Work out the finished part from the listing and answer in its coordinate system (mm). Round coordinates to 2 decimals unless told otherwise and drop trailing zeros. Loops run counter-clockwise (first coordinate to the right, second up) from the corner with the lowest first, then second, coordinate; pieces in that order, holes last. Notation, with made-up numbers: M 42.25,-4.5 L 80.25,-4.5 A18 cw 80.25,5.5 Z; hole C -39.75,-11.5 d11. An arc over 180 degrees is marked long. One line per item, written item: value.
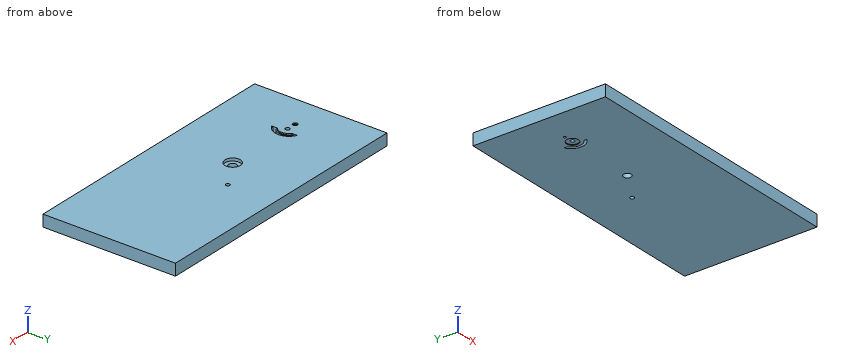
Autodesk Inventor part; units mm, degrees
ref_plane "Plano de trabajo1" through (-95, 0, 0) normal (0, 0, -1) x (-1, 0, 0)
ref_plane "YZ Plane" through (0, 0, 0) normal (1, 0, 0) x (0, 1, 0)
ref_plane "XZ Plane" through (0, 0, 0) normal (0, 1, 0) x (-1, 0, 0)
sketch "Boceto2" plane through (0, 0, 0) normal (0, 0, 1) x (1, 0, 0)
  line L0 (130, -85) -> (-130, -85)
  line L1 (-130, -85) -> (-130, 85)
  line L2 (-130, 85) -> (130, 85)
  line L3 (130, 85) -> (130, -85)
  line L4 (130, -85) -> (-130, 85) construction
  line L5 (-130, -85) -> (130, 85) construction
  point P0 (0, 0)
  dimension "d0" = 260
  dimension "d1" = 170
extrude "Extrusión1" add sketch "Boceto2" along normal blind 15
sketch "Boceto3" plane through (0, 0, 15) normal (0, 0, 1) x (1, 0, 0)
  line L0 (-95, 0) -> (-4.19, 0) construction
  circle A0 centre (-95, 0) radius 2.625
  circle A1 centre (-4.19, 0) radius 9.875
  line L1 (-130, 85) -> (-130, -85)
  line L2 (130, -85) -> (130, 85)
  line L3 (-130, -85) -> (130, -85)
  line L4 (130, 0) -> (80, 0) construction
  line L5 (80, 0) -> (80, -23.2237) construction
  arc A2 (-102.5, -15.9496) -> (-102.5, 15.9496) centre (-109.9995, 0) ccw
  arc A3 (-102.5, -9.8973) -> (-102.5, 9.8973) centre (-109.9995, 0) ccw
  line L6 (-95, 0) -> (-102.5, 0)
  line L7 (-102.5, 15.9496) -> (-102.5, 12.8966)
  line L8 (-102.5, 15.9496) -> (-102.5, 9.8973)
  line L9 (-102.5, -9.8973) -> (-102.5, -15.9496)
  point P0 (0, 0)
  point P1 (-130, 0)
  point P2 (-92.375, 0)
  point P3 (-97.5893, -0.4312)
  point P4 (-97.5893, 0.4312)
  dimension "d7" = 5.25
  dimension "d8" = 19.75
  dimension "d14" = 85
  dimension "d29" = 50
  dimension "d31" = 35
  dimension "d32" = 134.19
  dimension "d139" = 125.81
  dimension "d141" = 7.5
sketch "Boceto5" plane through (0, 0, 0) normal (0, 0, -1) x (-1, 0, 0)
  line L0 (-130, -85) -> (-130, 85)
  line L1 (130, -85) -> (-130, -85)
  line L2 (-130, -85) -> (-130, 85)
  line L3 (-130, 85) -> (130, 85)
  line L4 (130, 85) -> (130, -85)
  line L5 (130, -85) -> (-130, 85) construction
  line L6 (-130, -85) -> (130, 85) construction
  line L7 (119.5, 74.5) -> (-119.5, 74.5)
  line L8 (-119.5, 74.5) -> (-119.5, -74.5)
  line L9 (-119.5, -74.5) -> (119.5, -74.5)
  line L10 (119.5, -74.5) -> (119.5, 74.5)
  circle A0 centre (95, 0) radius 2.625
  circle A1 centre (95, 0) radius 2.625
  point P0 (0, 0)
  dimension "d23" = 10.5
  dimension "d25" = 5.25
sketch "Boceto6" plane through (0, 0, 15) normal (0, 0, 1) x (1, 0, 0)
  circle A0 centre (-4.19, 0) radius 10.125
  line L0 (-4.19, 0) -> (35.81, 0)
  line L1 (35.81, 0) -> (35.81, 25)
  circle A1 centre (35.81, 25) radius 2.5
  point P0 (0, 0)
  dimension "d35" = 40
  dimension "d36" = 25
  dimension "d152" = 5
ref_plane "Plano de trabajo4" through (0, 0, -4) normal (0, 0, -1) x (-1, 0, 0)
sketch "Boceto10" plane through (0, 0, -4) normal (0, 0, -1) x (-1, 0, 0)
  circle A0 centre (95, 0) radius 2.625
  circle A1 centre (95, 0) radius 7.5
  point P0 (0, 0)
  dimension "d51" = 15
ref_plane "Plano de trabajo1" through (-95, 0, 0) normal (0, 0, -1) x (-1, 0, 0)
sketch "Boceto12" plane through (0, 0, 15) normal (0, 0, 1) x (1, 0, 0)
  circle A0 centre (-95, 0) radius 2.625 construction
  circle A1 centre (-95, 0) radius 7.5 construction
  line L0 (-95, 0) -> (-82.5, 0) construction
  circle A2 centre (-82.5, 0) radius 3
  line L1 (-95, 0) -> (-107.5, 0) construction
  circle A3 centre (-107.5, 0) radius 3
  circle A4 centre (-107.5, 0) radius 1.5 construction
  circle A5 centre (-82.5, 0) radius 1.5 construction
  line L2 (-82.5, 0) -> (-97.5, 0) construction
  line L3 (-97.5, 0) -> (-97.5, 18.5) construction
  arc A6 (-89.1168, -15.9286) -> (-89.9998, 16.363) centre (-97.5, 0) ccw
  arc A7 (-89.9998, -16.2295) -> (-89.1168, -15.9286) centre (-90.514, -13.2739) ccw
  arc A8 (-89.9998, -16.2295) -> (-89.1168, -15.9286) centre (-90.514, -13.2739) ccw
  arc A9 (-92.595, 10.9517) -> (-92.4052, 10.8647) centre (-91.2508, 13.6338) ccw
  arc A10 (-89.9998, -16.2295) -> (-89.1168, -15.9286) centre (-90.514, -13.2739) ccw
  arc A11 (-89.8154, -14.6013) -> (-90, 14.6969) centre (-97.5, 0) ccw
  arc A12 (-89.9998, -11.2249) -> (-90, 11.225) centre (-97.5, 0) ccw
  arc A13 (-89.9998, -14.683) -> (-89.8154, -14.6013) centre (-90.514, -13.2739) ccw
  circle A14 centre (-82.5, 0) radius 1.5
  line L4 (-130, 85) -> (-130, -85)
  line L5 (-130, -85) -> (130, -85)
  line L6 (-82.5, 0) -> (-90, 0) construction
  line L7 (-90, 0) -> (-90, 18.2385) construction
  line L8 (-89.9998, 16.363) -> (-89.9998, -17.0131)
  arc A15 (-89.9998, -9.3674) -> (-90, 9.3675) centre (-97.5, 0) ccw
  arc A16 (-92.4052, 10.8647) -> (-92.6345, 10.9694) centre (-97.5, 0) ccw
  point P0 (0, 0)
  point P1 (-89.8154, -14.6013)
  point P2 (-91.2126, -11.9465)
  point P3 (-84.225, -2.4545)
  point P4 (-79.5, 0)
  point P5 (-81.225, -2.7156)
  point P6 (-84.225, 2.4545)
  point P7 (-81.225, 2.7156)
  point P8 (-84, 0)
  point P9 (-81, 0)
  point P10 (-89.9998, 11.2249)
  point P11 (-89.9998, 9.3674)
  point P12 (-85.5, 0)
  point P13 (-89.9998, 14.6969)
  dimension "d59" = 15
  dimension "d60" = 12.5
  dimension "d61" = 6
  dimension "d62" = 12.5
  dimension "d63" = 6
  dimension "d64" = 3
  dimension "d65" = 3
  dimension "d126" = 15
  dimension "d127" = 6
  dimension "d128" = 6
  dimension "d129" = 1.5
  dimension "d130" = 1.5
  dimension "d135" = 3
extrude "Extrusión10" cut sketch "Boceto12" against normal blind 1.5 contours A2 A11 | A11 A14 A12 A2 | A2 A12 A14 A11 | A12 A2 | A14 | A3
sketch "Boceto13" plane through (-82.5, 0, 13.5) normal (0, 0, 1) x (1, 0, 0)
  circle A0 centre (0, 0) radius 1.5
  circle A1 centre (-25, 0) radius 3
  circle A2 centre (-25, 0) radius 1.5
  point P0 (82.5, 0)
  dimension "d68" = 3
  dimension "d69" = 3
extrude "Extrusión11" cut sketch "Boceto13" against normal through all contours A0 | A2
extrude "Extrusión12" cut sketch "Boceto10" against normal blind 5
ref_plane "Plano de trabajo2" through (-4.19, 0, 15) normal (0, 0, 1) x (1, 0, 0)
sketch "Boceto15" plane through (-4.19, 0, 15) normal (0, 0, 1) x (1, 0, 0)
  circle A0 centre (0, 0) radius 5
  circle A1 centre (0, 0) radius 74 construction
  circle A2 centre (-90.81, 0) radius 2.625 construction
  circle A3 centre (-90.81, 0) radius 20 construction
  point P0 (4.19, 0)
  dimension "d77" = 10
  dimension "d80" = 148
  dimension "d82" = 40
extrude "Extrusión14" cut sketch "Boceto15" against normal through all
ref_plane "Plano de trabajo3" through (0, 0, -4) normal (0, 0, -1) x (-1, 0, 0)
sketch "Boceto17" plane through (0, 0, 15) normal (0, 0, 1) x (1, 0, 0)
  circle A0 centre (-95, 0) radius 2.625 construction
  circle A1 centre (-4.19, 0) radius 5 construction
  circle A2 centre (-4.19, 0) radius 40
  circle A3 centre (-4.19, 0) radius 15
  point P0 (0, 0)
  dimension "d87" = 80
  dimension "d88" = 30
sketch "Boceto20" plane through (0, 0, 15) normal (0, 0, 1) x (1, 0, 0)
  line L0 (130, 85) -> (-130, 85)
  line L1 (130, -85) -> (130, 85)
  line L2 (130, 85) -> (220, 85)
  line L3 (220, 85) -> (220, -85)
  line L4 (220, -85) -> (130, -85)
  line L5 (130, -85) -> (130, 85)
  point P0 (0, 0)
  dimension "d115" = 90
extrude "Extrusión22" add sketch "Boceto20" against normal blind 15
extrude "Extrusión23" cut sketch "Boceto3" against normal through all contours A0 A3 | A3 L6 A0 | A0 L6 A3
extrude "Extrusión24" [suppressed]
extrude "Extrusión25" cut sketch "Boceto12" against normal blind 1.5 contours A2 A11 | A6 A7 L8 A13 A11 A2 | A2 A11 L8 A6 | A12 A2 | A2 A15 L8 A12 | A12 L8 A15 A2
extrude "Extrusión26" cut sketch "Boceto12" against normal through all contours A11 A14 A12 A2 | A2 A12 L8 A11 | A11 A13 L8 A12 A2 | A2 A12 A14 A11
sketch "Boceto21" plane through (0, 0, 15) normal (0, 0, 1) x (1, 0, 0)
  line L0 (-130, 85) -> (-150, 85)
  line L1 (-150, 85) -> (-150, -85)
  line L2 (-150, -85) -> (-130, -85)
  line L3 (-130, -85) -> (-130, 85)
  line L4 (220, 85) -> (-130, 85)
  line L5 (-130, -85) -> (220, -85)
  line L6 (220, 85) -> (200, 85)
  line L7 (200, 85) -> (200, -85)
  line L8 (200, -85) -> (220, -85)
  line L9 (220, -85) -> (220, 85)
  point P0 (0, 0)
  dimension "d146" = 20
  dimension "d147" = 20
extrude "Extrusión28" add sketch "Boceto21" against normal blind 15 contours L3 L2 L1 L0
extrude "Extrusión29" cut sketch "Boceto21" against normal through all contours L4 L9 L5 L7
extrude "Extrusión30" cut sketch "Boceto6" against normal through all contours A1
extrude "Extrusión31" cut sketch "Boceto3" against normal blind 3.5 contours A1
properties part number "Cover"
1) Find the intervals of material crossed by probe 1 along X at (y, z) = (25, 3.25); probe 2 along Y at (x, z) = (-4.19, 12.25) (3 decimals); probe 3 along Y at (x, z) = (-95, 0.5), in increasing order. Write a range as from..to.
Check values:
probe 1: -150..33.31, 38.31..200
probe 2: -85..-9.875, 9.875..85
probe 3: -85..-7.5, 7.5..85
2) Find section A-A (x = -4.19). Give the vertices of the cut face in (y, z) (3 decimals).
Check values:
outline: M -85,0 L -5,0 L -5,11.5 L -9.875,11.5 L -9.875,15 L -85,15 Z; M 5,0 L 85,0 L 85,15 L 9.875,15 L 9.875,11.5 L 5,11.5 Z
3) Each of these flat-tipped pins is pushed along its axis until it touches: pin 1 (24 mm diameter, centred on x = -95, y = 0, fed in from -Z); pin 2 (5 mm diameter, centred on x = -107.5, y = 0, fed in from +Z). Where does it stop, or does it pass through?
Check values:
pin 1: z = 0
pin 2: z = 13.5
